from build123d import *

# Parameters (mm, degrees)
F0_R     = 10.975
F1_DEPTH = 3.5
F2_SIZE  = 0.5


with BuildPart() as f1:
    # F0 (on Top) → F1 (new body, symmetric)
    with BuildSketch(Plane.XY):
        with BuildLine():
            Line((12.5, -23.5), (12.5, 23.5))
            ThreePointArc((12.5, 23.5), (0, 36), (-12.5, 23.5))
            Line((-12.5, 23.5), (-12.5, -23.5))
            ThreePointArc((-12.5, -23.5), (0, -36), (12.5, -23.5))
        make_face()
        with Locations((0, -23.5)):
            Circle(F0_R, mode=Mode.SUBTRACT)
        Circle(F0_R, mode=Mode.SUBTRACT)
        with Locations((0, 23.5)):
            Circle(F0_R, mode=Mode.SUBTRACT)
    extrude(amount=F1_DEPTH, both=True)

    # F2
    f2_edges = [f1.edges().sort_by_distance(p)[0] for p in [
        (12.5, 0, -3.5),
        (0, 36, -3.5),
        (-12.5, 0, -3.5),
        (0, -36, -3.5),
        (-10.975, -23.5, -3.5),
        (-10.975, 0, -3.5),
        (-10.975, 23.5, -3.5),
        (12.5, 0, 3.5),
        (0, 36, 3.5),
        (-12.5, 0, 3.5),
        (0, -36, 3.5),
        (-10.975, -23.5, 3.5),
        (-10.975, 0, 3.5),
        (-10.975, 23.5, 3.5),
    ]]
    chamfer(f2_edges, length=F2_SIZE)


solid = f1.part
Read the model definition and answer for the solid it produces. Units are mm, in the model's axes. Coordinates: 2 decimals unless noted, no trailing zeros. Order: outer loops, then holes, each group sorted by start corner. A loop starts at its lowest first (then second) coordinate and runs counter-clockwise, first axis right, second up. Notation, with made-up numbers: M 63,-13 L 106,-13 A31 cw 106,25 Z; hole C 79.5,64 d3. An arc over 180 degrees is marked long. Put each result on its own line as item: value. Start each with the question number.
Item 1: The mould has two halves that part along X. Classify faces 1 (the face through (0, -36, 0)), 2 (the face through (-1.43, -12.62, -0.04)), 3 (the face through (-5, 11, 3.5)), 4 (the face through (-1.43, 10.88, -0.04)): +X half, -X half, draft (parallel to the pull), parting line (faces both ways), or undercut.
Item 2: Section C-C, the plane y = 0 is taken. Determine the outline of the cut face in (x, z) (3 decimals), plus the area to 4 significant figures.
Item 3: Given pin 1 Ø4 at (x, z) = (5.5, 1) entering from -Y; pin 2 Ø2 at (x, z) = (-4.5, 1) entering from +Y; pin 3 Ø1.5 at (x, z) = (-1.5, 2.5) entering from -Y, each flat-ended and moving along its own axis, determine where each tip first touches the part or whether it passes through.
Item 4: Consider probe 1 along Y at (x, z) = (0, 0.25) (3 decimals); probe 2 along Y at (x, z) = (-9.25, 0); probe 3 along X at (y, z) = (-16.5, 2). Determine where each line is inside the solid, lowest interval first. Write a range as [from, to].
Item 5: Section A-A, the plane x = 0 is taken. Count the separate pieces of the cut face and the enclosed holes in it, plus the area to 4 significant figures.
Item 6: Section B-B, the plane z = 1.5 is taken. Determine the outline of the cut face in (x, y) (3 decimals), plus the area to 3 significant figures.
Computed:
1. face 1: parting line
1. face 2: undercut
1. face 3: draft
1. face 4: undercut
2. outline: M -12.5,-3 L -12,-3.5 L -11.475,-3.5 L -10.975,-3 L -10.975,3 L -11.475,3.5 L -12,3.5 L -12.5,3 Z; M 10.975,-3 L 11.475,-3.5 L 12,-3.5 L 12.5,-3 L 12.5,3 L 12,3.5 L 11.475,3.5 L 10.975,3 Z
2. area: 20.35 mm2
3. pin 1: stops at y = -35.5
3. pin 2: stops at y = 35.5
3. pin 3: stops at y = -35.98
4. probe 1: y = [-36, -34.475], [-12.525, -10.975], [10.975, 12.525], [34.475, 36]
4. probe 2: y = [-31.91, -29.41], [-17.59, -5.91], [5.91, 17.59], [29.41, 31.91]
4. probe 3: x = [-12.5, -8.45], [8.45, 12.5]
5. separate pieces: 4
5. enclosed holes: 0
5. area: 41.05 mm2
6. outline: M -12.5,-23.5 A12.5 ccw 12.5,-23.5 L 12.5,23.5 A12.5 ccw -12.5,23.5 Z; hole C 0,-23.5 d21.95; hole C 0,0 d21.95; hole C 0,23.5 d21.95
6. area: 531 mm2
